Source: CAD feature listing. Evaluate the final solid. Frame: model axes, mm. A direction names the side the tool comes from. Round coordinates to 2 decimals unless told otherwise and drop trailing zeros. Write each loop counter-clockwise with the first axis right and the second up, starting at its lowest first coordinate (ties: lowest second). Pieces come first, ordered by that corner, then holes. Notation, with made-up numbers: M 31,38.25 L 86,38.25 A29 cw 86,77.25 Z; hole C 58.25,-27.75 d1. An arc over 180 degrees is marked long. Answer in a Markdown table with one row per item. Add a question column.
Item 1: Cut plane D-D on x = 4.5. Return loops of the section in (y, z), and give its area (3 significant figures).
Item 2: Cut plane A-A on z = 0.9. Return loops of the section in (x, y).
Item 3: Contact query for flat-ended pins moving along their axis: pin 1 (3 mm diameter, centred on x = -9, y = -2.5, fed in from -Z); pin 2 (0.9 mm diameter, centred on x = 6, z = 1, fed in from +Y); pin 3 (0.9 mm diameter, centred on x = -14, z = 2, fed in from -Y); pin 4 (1.5 mm diameter, centred on y = -8.5, z = 2.5, fed in from +X). Output: stop coordinate, or through.
Item 4: Material intervals for probe 1 along Y at (x, z) = (-10, 1.2); probe 2 along Y at (x, z) = (-13.5, 0.4); probe 3 along X at (y, z) = (-3, 2.55), sorted ascending.
Item 5: Mould query, pull axis X, two halves, no side actions, for faces 1 (the face through (-10, 12, 1)), 2 (the face through (-10, -11, 1)), 3 (the face through (-10, 9, 1)), 4 (the face through (6, 10, 1)). Classes: released by +X, released by -X, zero draft, split by the parting line, or undercut.
Item 6: Set-up query: faces 5 (the face through (20, -6, 1)), 6 (the face through (-16, -10, 1)), 7 (the face through (-16, 10, 1)), 8 (the face through (20, 6, 1)). Return all of +Z, -Z, +X, -X, +Y, -Y with unobstructed straight access to the full face (end or side cutting, diameter ignored); none if empty.
Item 7: Cut plane C-C on y = -3. Return loops of the section in (x, z), and give its area (3 significant figures).
Item 8: Cut plane B-B on x = -10. Return loops of the section in (y, z), and give its area (3 significant figures).
Autodesk Inventor part; units mm, degrees
ref_plane "YZ Plane" through (0, 0, 0) normal (1, 0, 0) x (0, 1, 0)
ref_plane "XZ Plane" through (0, 0, 0) normal (0, 1, 0) x (-1, 0, 0)
ref_plane "XY Plane" through (0, 0, 0) normal (0, 0, 1) x (1, 0, 0)
sketch "Sketch1" plane through (0, 0, 0) normal (0, 0, 1) x (1, 0, 0)
  line L0 (-20, -10) -> (-20, 10)
  circle A0 centre (20, 0) radius 1
  arc A1 (20, -2) -> (20, 2) centre (20, 0) ccw
  line L1 (20, 10) -> (20, 2)
  line L2 (20, -2) -> (20, -10)
  circle A2 centre (-10, -10) radius 1
  arc A3 (-12, -10) -> (-8, -10) centre (-10, -10) ccw
  circle A4 centre (-10, 10) radius 1
  arc A5 (-8, 10) -> (-12, 10) centre (-10, 10) ccw
  line L3 (20, -10) -> (-8, -10)
  line L4 (-12, -10) -> (-20, -10)
  line L5 (-10, -10) -> (-9, -10)
  line L6 (-8, -10) -> (20, -10)
  line L7 (-20, 10) -> (-12, 10)
  line L8 (-8, 10) -> (20, 10)
  point P0 (0, 0)
  dimension "d8" = 2
  dimension "d0" = 20
  dimension "d1" = 40
  dimension "d4" = 2
  dimension "d5" = 4
  dimension "d6" = 0
  dimension "d7" = 10
  dimension "d9" = 4
  dimension "d10" = 2
  dimension "d11" = 4
extrude "Extrusion1" add sketch "Sketch1" along normal blind 3
properties part number "current sensor"
Results below:
| question | item | result |
|---|---|---|
| 1 | outline | M -10,0 L 10,0 L 10,3 L -10,3 Z |
| 1 | area | 60.0 mm2 |
| 2 | outline | M -20,-10 L -12,-10 A2 ccw -8,-10 L 20,-10 L 20,-2 A2 ccw 20,2 L 20,10 L -8,10 A2 ccw -12,10 L -20,10 Z; hole C -10,-10 d2; hole C -10,10 d2; hole C 20,0 d2 |
| 3 | pin 1 | z = 0 |
| 3 | pin 2 | y = 10 |
| 3 | pin 3 | y = -10 |
| 3 | pin 4 | x = 20 |
| 4 | probe 1 | -12 to -11, -9 to 9, 11 to 12 |
| 4 | probe 2 | -10 to 10 |
| 4 | probe 3 | -20 to 20 |
| 5 | face 1 | split by the parting line |
| 5 | face 2 | undercut |
| 5 | face 3 | undercut |
| 5 | face 4 | zero draft |
| 6 | face 5 | +Z, -Z, +X, -Y |
| 6 | face 6 | +Z, -Z, -X, -Y |
| 6 | face 7 | +Z, -Z, -X, +Y |
| 6 | face 8 | +Z, -Z, +X, +Y |
| 7 | outline | M -20,0 L 20,0 L 20,3 L -20,3 Z |
| 7 | area | 120 mm2 |
| 8 | outline | M -12,0 L -11,0 L -11,3 L -12,3 Z; M -9,0 L 9,0 L 9,3 L -9,3 Z; M 11,0 L 12,0 L 12,3 L 11,3 Z |
| 8 | area | 60.0 mm2 |
